from build123d import *

# Parameters (mm, degrees)
SKETCH18_R            = 148.43125
BOSS_EXTRUDE1_DEPTH   = 6.35
F_6_CLEARANCE_HOLE1_D = 3.7973
CUT_EXTRUDE1_DEPTH    = 6.35
F_6_CLEARANCE_HOLE2_D = 3.7973
SKETCH29_W            = 44.45
SKETCH29_H            = 60.325
CUT_EXTRUDE2_DEPTH    = 7.35
SKETCH30_R            = 12.7
SKETCH30_W            = 22.225
SKETCH30_H            = 30.1625
CUT_EXTRUDE3_DEPTH    = 6.35
F_6_CLEARANCE_HOLE3_D = 3.7973


with BuildPart() as part:
    # Sketch18 → Boss-Extrude1 (new body)
    with BuildSketch(Plane(origin=(0, 0, 0), x_dir=(1, 0, 0), z_dir=(0, 1, 0))):
        Circle(SKETCH18_R)
    extrude(amount=BOSS_EXTRUDE1_DEPTH)

    # #6 Clearance Hole1 (through all)
    with Locations(Plane(origin=(0, 6.35, 0), x_dir=(1, 0, 0), z_dir=(0, 1, 0))):
        with Locations((-101.6, 101.6), (101.6, 101.6), (101.6, -101.6), (-101.6, -101.6), (-124.434078933, 71.842048969), (-71.842048969, -124.434078933), (124.434078933, -71.842048969), (71.842048969, 124.434078933)):
            Hole(F_6_CLEARANCE_HOLE1_D / 2)

    # Sketch23 → Cut-Extrude1 (cut)
    with BuildSketch(Plane(origin=(0, 6.35, 0), x_dir=(1, 0, 0), z_dir=(0, 1, 0))):
        with BuildLine():
            ThreePointArc((-72.791373969, -126.078358066), (-73.486328101, -123.484753933), (-70.892723969, -122.7897998))
            ThreePointArc((-70.892723969, -122.7897998), (-86.313511899, -112.485958726), (-100.25745171, -100.25745171))
            ThreePointArc((-100.25745171, -100.25745171), (-99.845876126, -100.873418101), (-99.70135, -101.6))
            ThreePointArc((-99.70135, -101.6), (-100.873418101, -103.354123874), (-102.94254829, -102.94254829))
            ThreePointArc((-102.94254829, -102.94254829), (-88.625161673, -115.498559365), (-72.791373969, -126.078358066))
        make_face()
        with BuildLine():
            ThreePointArc((-100.25745171, 100.25745171), (-102.94254829, 100.25745171), (-102.94254829, 102.94254829))
            ThreePointArc((-102.94254829, 102.94254829), (-115.498559365, 88.625161673), (-126.078358066, 72.791373969))
            ThreePointArc((-126.078358066, 72.791373969), (-123.942672153, 73.676004039), (-122.535428933, 71.842048969))
            ThreePointArc((-122.535428933, 71.842048969), (-122.600123863, 71.350642189), (-122.7897998, 70.892723969))
            ThreePointArc((-122.7897998, 70.892723969), (-112.485958726, 86.313511899), (-100.25745171, 100.25745171))
        make_face()
        with BuildLine():
            ThreePointArc((100.25745171, 100.25745171), (100.25745171, 102.94254829), (102.94254829, 102.94254829))
            ThreePointArc((102.94254829, 102.94254829), (88.625161673, 115.498559365), (72.791373969, 126.078358066))
            ThreePointArc((72.791373969, 126.078358066), (73.486328101, 125.383403933), (73.740698969, 124.434078933))
            ThreePointArc((73.740698969, 124.434078933), (72.791373969, 122.7897998), (70.892723969, 122.7897998))
            ThreePointArc((70.892723969, 122.7897998), (86.313511899, 112.485958726), (100.25745171, 100.25745171))
        make_face()
        with BuildLine():
            ThreePointArc((126.078358066, -72.791373969), (123.484753933, -73.486328101), (122.7897998, -70.892723969))
            ThreePointArc((122.7897998, -70.892723969), (112.485958726, -86.313511899), (100.25745171, -100.25745171))
            ThreePointArc((100.25745171, -100.25745171), (102.326581899, -99.845876126), (103.49865, -101.6))
            ThreePointArc((103.49865, -101.6), (103.354123874, -102.326581899), (102.94254829, -102.94254829))
            ThreePointArc((102.94254829, -102.94254829), (115.498559365, -88.625161673), (126.078358066, -72.791373969))
        make_face()
    extrude(amount=-CUT_EXTRUDE1_DEPTH, mode=Mode.SUBTRACT)

    # #6 Clearance Hole2 (through all)
    with Locations(Plane(origin=(0, 6.35, 0), x_dir=(1, 0, 0), z_dir=(0, 1, 0))):
        with Locations((57.15, -45.24375), (57.15, -88.10625), (100.0125, -88.10625), (100.0125, -45.24375), (-28.575, -63.5), (28.575, -63.5), (-28.575, 127), (28.575, 127)):
            Hole(F_6_CLEARANCE_HOLE2_D / 2)

    # Sketch29 → Cut-Extrude2 (cut, through all)
    with BuildSketch(Plane(origin=(0, 6.35, 0), x_dir=(1, 0, 0), z_dir=(0, 1, 0))):
        with Locations((0, -42.8625)):
            Rectangle(SKETCH29_W, SKETCH29_H)
    extrude(amount=-CUT_EXTRUDE2_DEPTH, mode=Mode.SUBTRACT)

    # Sketch30 → Cut-Extrude3 (cut)
    with BuildSketch(Plane(origin=(0, 6.35, 0), x_dir=(1, 0, 0), z_dir=(0, 1, 0))):
        with Locations((-80.82230509, 80.82230509)):
            Circle(SKETCH30_R)
        with Locations((80.82230509, 80.82230509)):
            Circle(SKETCH30_R)
        with Locations((-80.82230509, -80.82230509)):
            Circle(SKETCH30_R)
        with Locations((-44.30980509, -111.77855509)):
            Rectangle(SKETCH30_W, SKETCH30_H)
    extrude(amount=-CUT_EXTRUDE3_DEPTH, mode=Mode.SUBTRACT)

    # #6 Clearance Hole3 (through all)
    with Locations(Plane(origin=(0, 6.35, 0), x_dir=(1, 0, 0), z_dir=(0, 1, 0))):
        with Locations((-50.8, 101.6), (-76.2, 101.6), (-101.6, 76.2), (-50.8, 76.2), (-50.8, 50.8), (-76.2, 50.8), (-101.6, 50.8), (-127, 50.8), (-50.8, 25.4), (-76.2, 25.4), (-101.6, 25.4), (-127, 25.4), (-101.6, 0), (-127, 0), (-127, -25.4), (-101.6, -25.4), (-127, -50.8), (-101.6, -50.8), (-101.6, -76.2), (-76.2, -101.6), (-50.8, -76.2), (-76.2, -50.8), (-50.8, -50.8), (-50.8, -25.4), (-76.2, -25.4), (-76.2, 0), (-50.8, 0), (50.8, 101.6), (76.2, 101.6), (50.8, 76.2), (101.6, 76.2), (101.6, 50.8), (127, 50.8), (127, 25.4), (127, 0), (127, -25.4), (50.8, 50.8), (50.8, 25.4), (50.8, 0), (50.8, -25.4), (76.2, -25.4), (101.6, -25.4), (101.6, 0), (76.2, 0), (76.2, 25.4), (76.2, 50.8), (101.6, 25.4), (127, -50.8), (76.2, -101.6), (50.8, -101.6), (-25.4, -101.6), (25.4, -101.6), (25.4, -127), (50.8, -127), (-25.4, -127)):
            Hole(F_6_CLEARANCE_HOLE3_D / 2)


solid = part.part
Here's how the part is built. I have some questions about the finished solid (model axes, mm). A direction names the side the tool comes from. Round coordinates to 2 decimals unless told otherwise and drop trailing zeros. Order: outer loops, then holes, each group sorted by start corner. A loop starts at its lowest first (then second) coordinate and runs counter-clockwise, first axis right, second up. Notation, with made-up numbers: M 61,41.5 L 117,41.5 A21 cw 117,58.5 Z; hole C 81,-28 d2. An arc over 180 degrees is marked long. Return JSON: item names as keys, results as strings. Group by question number.
1. If we mould it in two halves opening along X, with no side actions, what happens to faces 1 (the face through (-68.71, 3.22, -84.64)), 2 (the face through (-32.18, 3.13, 144.9)), 3 (the face through (-2, 0, -2))? For each: pulls with the +X half, pulls with the -X half, needs draft (parallel to the pull), parting line crosses it, or undercut.
2. I'm going to push flat-ended pins straight in: pin 1 Ø4.5 at (x, z) = (100.01, 88.11) entering from +Y; pin 2 Ø1.5 at (y, z) = (4, -27.5) entering from +X; pin 3 Ø2 at (y, z) = (5, 95) entering from -X; pin 4 Ø1.9 at (y, z) = (4, 113) entering from +X. Where does each tip first touch, or does it pass through?
3. If we section it at A-A on z = 19: List the corners of the cut face in (x, y) for me (3 decimals), then the cut area to 3 significant figures.
4. If we section it at B-B on z = -110: List the corners of the cut face in (x, y) for me.
5. On a 3-axis mill with a long thin cutter (end or side, diameter ignored), from which of +Z, -Z, +X, -X, +Y, -Y can I reach the whole of each face in a straight line? I mean faces 4 (the face through (-2, 6.35, -2)), 5 (the face through (0, 3, 12.7)). Say none if no direction works.
6. If we section it at C-C on y = 5.25: State how many separate pieces and enclosed holes the cut face has, then the cut area to 3 significant figures.
7. If we section it at D-D on z = -59: List the corners of the cut face in (x, y) for me.
8. Please list where these lines run through material, in increasing order: probe 1 along Z at (x, y) = (3, 4.5) (3 decimals); probe 2 along Z at (x, y) = (127.5, 4.75); probe 3 along Z at (x, y) = (-127, 2.25).
Reply:
{
 "1": {"face 1": "undercut", "face 2": "parting line crosses it", "face 3": "needs draft"},
 "2": {"pin 1": "y = 6.35", "pin 2": "x = 146", "pin 3": "x = -114.87", "pin 4": "x = 97.35"},
 "3": {"outline": "M -147.21,0 L -22.225,0 L -22.225,6.35 L -147.21,6.35 Z; M 22.225,0 L 147.21,0 L 147.21,6.35 L 22.225,6.35 Z", "area": "1,590 mm^2"},
 "4": {"outline": "M -99.66,0 L 89.46,0 L 89.46,6.35 L -99.66,6.35 Z; M 95.36,0 L 99.66,0 L 99.66,6.35 L 95.36,6.35 Z"},
 "5": {"face 4": "+Z, -Z, +X, -X, +Y", "face 5": "+Y, -Y"},
 "6": {"separate pieces": "1", "enclosed holes": "72", "area": "63,000 mm^2"},
 "7": {"outline": "M -136.2,0 L 136.2,0 L 136.2,6.35 L -136.2,6.35 Z"},
 "8": {"probe 1": "-148.401 to 12.7, 73.025 to 148.401", "probe 2": "-76 to -52.63, -48.97 to -27.23, -23.57 to -1.83, 1.83 to 23.57, 27.23 to 48.97, 52.63 to 76", "probe 3": "-76.83 to -52.7, -48.9 to -27.3, -23.5 to -1.9, 1.9 to 23.5, 27.3 to 48.9, 52.7 to 76.83"}
}
